Can you work these out from the model? Positions are in its coordinate system, mm. A direction names the side the tool comes from. Coordinates: 2 decimals unless noted, no trailing zeros. Order: outer loops, then holes, each group sorted by start corner. A loop starts at its lowest first (then second) coordinate and runs counter-clockwise, first axis right, second up. Notation, with made-up numbers: (32, -18.75) -> (78, -18.75) arc R27 cw to (78, 11.25) -> close; hole circle Ø5 at (48.25, 49.5). An arc over 180 degrees is marked (long way). Answer in a Markdown table with one row per item. Add a question column.
1. If I drill on line 1 along X through (y, z) = (-65.9, 0); line 2 along X through (y, z) = (-28, 4.5); line 3 along Y through (x, z) = (-7, 7), over which ranges is the centre line in solid material (lowest first)? Write a range as [from, to].
2. Imagine slicing it at C-C on y = -44. Write out the boundary of the cut face in (x, z).
3. On a 3-axis mill with a long thin cutter (end or side, diameter ignored), from which of +Z, -Z, +X, -X, +Y, -Y can I reach the whole of each face in a straight line? I mean faces 1 (the face through (-2, -10, -2)), 2 (the face through (0, -4, -1.5)), 3 (the face through (-7.576, -14.717, 9.88)), 4 (the face through (-2.4, -65.4, -2.4)). Say none if no direction works.
4. Imagine slicing it at B-B on y = -18.5. Write out the boundary of the cut face in (x, z).
5. Will these pins go through, and if not, where does the flat tip stop? pin 1 (4 mm diameter, centred on y = -24.5, z = 5.5, fed in from -X); pin 2 (7 mm diameter, centred on x = 5, z = -5.5, fed in from -Y); pin 3 (1.8 mm diameter, centred on x = 0, z = 8.5, fed in from +Y).
from build123d import *
from build123d.topology import SkipClean

# Parameters (mm, degrees)
EXTRUDE_1_DEPTH     = 8
SKETCH_3_R          = 2
EXTRUDE_2_DEPTH     = 2
SKETCH_4_R          = 3.5
EXTRUDE_3_DEPTH     = 2.4
SKETCH_5_R          = 12.45
EXTRUDE_4_DEPTH     = 4.7
SKETCH_6_R          = 12.4495
EXTRUDE_5_DEPTH     = 14
SKETCH_7_R          = 12.45
EXTRUDE_6_DEPTH     = 4.3
SKETCH_8_R          = 12.1
EXTRUDE_7_DEPTH     = 31
SKETCH_9_R          = 11.6
CUT_EXTRUDE_3_DEPTH = 1
SKETCH_10_R         = 3
EXTRUDE_8_DEPTH     = 2
FILLET_1_R          = 1
SKETCH_11_R         = 1.5
CUT_EXTRUDE_4_DEPTH = 7


with BuildPart() as part:
    # Эскиз2 → Бобышка-Вытянуть1 (new body)
    with BuildSketch(Plane(origin=(0, 0, 0), x_dir=(1, 0, 0), z_dir=(0, 1, 0))):
        with BuildLine():
            Line((1.322875656, 1.5), (-1.322875656, 1.5))
            ThreePointArc((-1.322875656, 1.5), (-0.822875656, -1.822875656), (2, 0))
            ThreePointArc((2, 0), (1.822875656, 0.822875656), (1.322875656, 1.5))
        make_face()
    extrude(amount=-EXTRUDE_1_DEPTH)

    # Эскиз3 → Бобышка-Вытянуть2 (add)
    with BuildSketch(Plane(origin=(0, -8, 0), x_dir=(-1, 0, 0), z_dir=(0, -1, 0))):
        with Locations(Location((0, 0, 0), (0, 0, 48.590377891))):
            Circle(SKETCH_3_R)
    extrude(amount=EXTRUDE_2_DEPTH)

    # Эскиз4 → Бобышка-Вытянуть3 (add)
    with SkipClean():  # the faces are left unmerged after this step: merging them gives an invalid solid
        with BuildSketch(Plane(origin=(0, -10, 0), x_dir=(-1, 0, 0), z_dir=(0, -1, 0))):
            with Locations(Location((0, 0, 0), (0, 0, 90))):
                Circle(SKETCH_4_R)
        extrude(amount=EXTRUDE_3_DEPTH)

    # Эскиз5 → Бобышка-Вытянуть4 (add)
    with SkipClean():  # the faces are left unmerged after this step: merging them gives an invalid solid
        with BuildSketch(Plane(origin=(0, -12.4, 0), x_dir=(-1, 0, 0), z_dir=(0, -1, 0))):
            with Locations(Location((0, 0, 0), (0, 0, 90))):
                Circle(SKETCH_5_R)
        extrude(amount=EXTRUDE_4_DEPTH)

    # Эскиз6 → Бобышка-Вытянуть5 (add)
    with SkipClean():  # the faces are left unmerged after this step: merging them gives an invalid solid
        with BuildSketch(Plane(origin=(0, -17.1, 0), x_dir=(-1, 0, 0), z_dir=(0, -1, 0))):
            with Locations(Location((0, 0, 0), (0, 0, 90))):
                Circle(SKETCH_6_R)
        extrude(amount=EXTRUDE_5_DEPTH)

    # Эскиз7 → Бобышка-Вытянуть6 (add)
    with SkipClean():  # the faces are left unmerged after this step: merging them gives an invalid solid
        with BuildSketch(Plane(origin=(0, -31.1, 0), x_dir=(-1, 0, 0), z_dir=(0, -1, 0))):
            with Locations(Location((0, 0, 0), (0, 0, 90))):
                Circle(SKETCH_7_R)
        extrude(amount=EXTRUDE_6_DEPTH)

    # Эскиз8 → Бобышка-Вытянуть7 (add)
    with SkipClean():  # the faces are left unmerged after this step: merging them gives an invalid solid
        with BuildSketch(Plane(origin=(0, -35.4, 0), x_dir=(-1, 0, 0), z_dir=(0, -1, 0))):
            with Locations(Location((0, 0, 0), (0, 0, 90))):
                Circle(SKETCH_8_R)
        extrude(amount=EXTRUDE_7_DEPTH)

    # Эскиз9 → Вырез-Вытянуть3 (cut)
    with SkipClean():  # the faces are left unmerged after this step: merging them gives an invalid solid
        with BuildSketch(Plane(origin=(0, -66.4, 0), x_dir=(-1, 0, 0), z_dir=(0, -1, 0))):
            with Locations(Location((0, 0, 0), (0, 0, 90))):
                Circle(SKETCH_9_R)
        extrude(amount=-CUT_EXTRUDE_3_DEPTH, mode=Mode.SUBTRACT)

    # Эскиз10 → Бобышка-Вытянуть8 (add)
    with SkipClean():  # the faces are left unmerged after this step: merging them gives an invalid solid
        with BuildSketch(Plane(origin=(0, -65.4, 0), x_dir=(-1, 0, 0), z_dir=(0, -1, 0))):
            with Locations(Location((0, 0, 0), (0, 0, 90))):
                Circle(SKETCH_10_R)
        extrude(amount=EXTRUDE_8_DEPTH)

    # Скругление1
    fillet_1_edges = [part.edges().sort_by_distance(p)[0] for p in [
        (0, -67.4, 3),
    ]]
    fillet(fillet_1_edges, radius=FILLET_1_R)

    # Эскиз11 → Вырез-Вытянуть4 (cut)
    with SkipClean():  # the faces are left unmerged after this step: merging them gives an invalid solid
        with BuildSketch(Plane(origin=(0, -12.4, 0), x_dir=(1, 0, 0), z_dir=(0, 1, 0))):
            with Locations(Location((0, 8.5, 0), (0, 0, 270))):
                Circle(SKETCH_11_R)
            with Locations(Location((0, -8.5, 0), (0, 0, 270))):
                Circle(SKETCH_11_R)
        extrude(amount=-CUT_EXTRUDE_4_DEPTH, mode=Mode.SUBTRACT)


solid = part.part
Answers follow:
| question | item | result |
|---|---|---|
| 1 | line 1 | x = [-12.1, -11.6], [-3, 3], [11.6, 12.1] |
| 1 | line 2 | x = [-11.61, 11.61] |
| 1 | line 3 | y = [-65.4, -12.4] |
| 2 | outline | circle Ø24.2 at (0, 0) |
| 3 | face 1 | +Y |
| 3 | face 2 | -Z, +X, -X, +Y |
| 3 | face 3 | +Y, -Y |
| 3 | face 4 | -Y |
| 4 | outline | circle Ø24.9 at (0, 0); hole circle Ø3 at (0, -8.5); hole circle Ø3 at (0, 8.5) |
| 5 | pin 1 | stops at x = -11.95 |
| 5 | pin 2 | stops at y = -65.4 |
| 5 | pin 3 | stops at y = -19.4 |
